Geometry: final body of the model. Coordinates: model frame, mm. Face numbers are marked on the shaded views. A direction names the side the tool comes from. Round coordinates to 2 decimals unless told otherwise and drop trailing zeros. Order: outer loops, then holes, each group sorted by start corner. A loop starts at its lowest first (then second) coordinate and runs counter-clockwise, first axis right, second up. Notation, with made-up numbers: M 31.25,53.5 L 47.25,53.5 A32 cw 47.25,90.5 Z; hole C 13,-18.75 d3. An arc over 180 degrees is marked long. Put each result on its own line as item: value. Start each with the question number.
1) Section D-D, the plane x = 51. Return loops of the section in (y, z), then the cut area to 3 significant figures.
2) First-contact query: P1, Ø1.8, axis at x = 12, z = 4, coming from the -Y side; P2, Ø4, axis at x = 51, y = 61, coming from the +Z side. Flat tips, straight axial feed; report the tip coordinate or a pass-through.
3) Section C-C, the plane y = 17. Return loops of the section in (x, z), then the cut area to 3 significant figures.
4) Access query for the marked faces 3 and 4. Directions: +Z, -Z, +X, -X, +Y, -Y. A direction counts if a zero-diameter tool reaches every point of the face in a straight line with its end or side. Return the directions, or none.
5) Section B-B, the plane y = 76. Return loops of the section in (x, z), then the cut area to 3 significant figures.
6) Section A-A, the plane y = 33.5. Return loops of the section in (x, z), then the cut area to 3 significant figures.
7) Draft query along X for the marked faces 1 and 2. Return one class per face: pulls with the +X half, pulls with the -X half, needs draft (parallel to the pull), parting line crosses it, or undercut.
8) Material intervals for probe 1 along X at (y, z) = (8.5, 5.2); probe 2 along Y at (x, z) = (27.5, 0.8); probe 3 along X at (y, z) = (36, 4.7), sorted ascending. Write a range as [from, to].
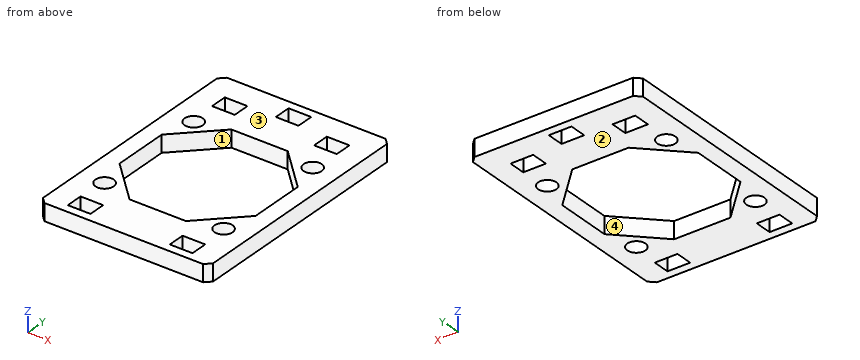
Autodesk Inventor part; units mm, degrees
ref_plane "YZ Plane" through (0, 0, 0) normal (1, 0, 0) x (0, 1, 0)
ref_plane "XZ Plane" through (0, 0, 0) normal (0, 1, 0) x (-1, 0, 0)
ref_plane "XY Plane" through (0, 0, 0) normal (0, 0, 1) x (1, 0, 0)
sketch "Sketch1" plane through (0, 0, 0) normal (0, 0, 1) x (1, 0, 0)
  line L0 (0, 0) -> (60, 0)
  line L1 (60, 0) -> (60, 86)
  line L2 (60, 86) -> (0, 86)
  line L3 (0, 86) -> (0, 0)
  line L4 (54, 30.0589) -> (39.9411, 16)
  line L5 (39.9411, 16) -> (20.0589, 16)
  line L6 (20.0589, 16) -> (6, 30.0589)
  line L7 (6, 30.0589) -> (6, 49.9411)
  line L8 (6, 49.9411) -> (20.0589, 64)
  line L9 (20.0589, 64) -> (39.9411, 64)
  line L10 (39.9411, 64) -> (54, 49.9411)
  line L11 (54, 49.9411) -> (54, 30.0589)
  line L12 (9, 61) -> (51, 61) construction
  line L13 (51, 61) -> (51, 19) construction
  line L14 (51, 19) -> (9, 19) construction
  line L15 (9, 19) -> (9, 61) construction
  circle A0 centre (9, 61) radius 3.2
  circle A1 centre (9, 19) radius 3.2
  circle A2 centre (51, 19) radius 3.2
  circle A3 centre (51, 61) radius 3.2
  line L16 (8, 9) -> (16, 9)
  line L17 (16, 9) -> (16, 3)
  line L18 (16, 3) -> (8, 3)
  line L19 (8, 3) -> (8, 9)
  line L20 (44, 9) -> (52, 9)
  line L21 (52, 9) -> (52, 3)
  line L22 (52, 3) -> (44, 3)
  line L23 (44, 3) -> (44, 9)
  line L24 (8, 77) -> (16, 77)
  line L25 (16, 77) -> (16, 71)
  line L26 (16, 71) -> (8, 71)
  line L27 (8, 71) -> (8, 77)
  line L28 (44, 77) -> (52, 77)
  line L29 (52, 77) -> (52, 71)
  line L30 (52, 71) -> (44, 71)
  line L31 (44, 71) -> (44, 77)
  line L32 (26, 83) -> (34, 83)
  line L33 (34, 83) -> (34, 77)
  line L34 (34, 77) -> (26, 77)
  line L35 (26, 77) -> (26, 83)
  line L36 (12, 71) -> (12, 9) construction
  point P0 (30, 40)
  point P1 (30, 61)
  point P2 (30, 64)
  point P3 (9, 40)
  point P4 (6, 40)
  point P5 (12, 40)
  point P6 (30, 77)
  dimension "d0" = 42
  dimension "d1" = 42
  dimension "d2" = 48
  dimension "d3" = 6.4
  dimension "d4" = 6.4
  dimension "d5" = 6.4
  dimension "d6" = 6.4
  dimension "d7" = 6
  dimension "d8" = 8
  dimension "d9" = 6
  dimension "d10" = 8
  dimension "d11" = 3
  dimension "d12" = 8
  dimension "d13" = 6
  dimension "d14" = 3
  dimension "d15" = 86
  dimension "d16" = 6
  dimension "d17" = 6
  dimension "d18" = 8
  dimension "d19" = 8
extrude "Extrusion1" add sketch "Sketch1" along normal blind 6
chamfer "Chamfer1" distance 2 angle 45 4 edges at (0, 0, 3) (60, 0, 3) (60, 86, 3) (0, 86, 3)
properties part number "x_iddler_c_mount"
Result sheet:
1. outline: M 0,0 L 3,0 L 3,6 L 0,6 Z; M 9,0 L 15.8,0 L 15.8,6 L 9,6 Z; M 22.2,0 L 27.06,0 L 27.06,6 L 22.2,6 Z; M 52.94,0 L 57.8,0 L 57.8,6 L 52.94,6 Z; M 64.2,0 L 71,0 L 71,6 L 64.2,6 Z; M 77,0 L 86,0 L 86,6 L 77,6 Z
1. area: 212 mm2
2. P1: stops at y = 0
2. P2: passes through
3. outline: M 0,0 L 6.5,0 L 6.5,6 L 0,6 Z; M 11.5,0 L 19.06,0 L 19.06,6 L 11.5,6 Z; M 40.94,0 L 48.5,0 L 48.5,6 L 40.94,6 Z; M 53.5,0 L 60,0 L 60,6 L 53.5,6 Z
3. area: 169 mm2
4. face 3: +Z, +X, -X, +Y, -Y
4. face 4: +Z, -Z
5. outline: M 0,0 L 8,0 L 8,6 L 0,6 Z; M 16,0 L 44,0 L 44,6 L 16,6 Z; M 52,0 L 60,0 L 60,6 L 52,6 Z
5. area: 264 mm2
6. outline: M 0,0 L 6,0 L 6,6 L 0,6 Z; M 54,0 L 60,0 L 60,6 L 54,6 Z
6. area: 72.0 mm2
7. face 1: undercut
7. face 2: needs draft
8. probe 1: x = [0, 8], [16, 44], [52, 60]
8. probe 2: y = [0, 16], [64, 77], [83, 86]
8. probe 3: x = [0, 6], [54, 60]
